from build123d import *

# Parameters (mm, degrees)
SKETCH016_W             = 35.6
SKETCH016_H             = 11.6
PAD009_DEPTH            = 0.8
SKETCH017_W             = 35.6
SKETCH017_H             = 11.6
SKETCH017_W_2           = 34
SKETCH017_H_2           = 10
PAD010_DEPTH            = 55.8
SKETCH018_W             = 6
SKETCH018_H             = 12
POCKET007_DEPTH         = 5.8
BODY005_PLACEMENT_ANGLE = 270


with BuildPart() as part:
    # Sketch016 → Pad009 (new body)
    with BuildSketch(Plane.XY):
        Rectangle(SKETCH016_W, SKETCH016_H)
    extrude(amount=PAD009_DEPTH)

    # Sketch017 → Pad010 (join)
    with BuildSketch(Plane.XY):
        Rectangle(SKETCH017_W, SKETCH017_H)
        Rectangle(SKETCH017_W_2, SKETCH017_H_2, mode=Mode.SUBTRACT)
    extrude(amount=PAD010_DEPTH)

    # Sketch018 (on Face5 of Pad010) → Pocket007 (cut)
    with BuildSketch(Plane.XZ.offset(5.8)):
        with Locations((14.8, 49.8)):
            Rectangle(SKETCH018_W, SKETCH018_H)
    extrude(amount=-POCKET007_DEPTH, mode=Mode.SUBTRACT)


with BuildPart() as part_1:
    # Body005 placement: moved
    add(part.part.moved(Location((-33.1, -35.587276, 51.887276))).rotate(Axis((-33.1, -35.587276, 51.887276), (1, 0, 0)), BODY005_PLACEMENT_ANGLE))


solid = part_1.part
Verification items for the finished model (mm, model axes). A direction names the side the tool comes from. Round coordinates to 2 decimals unless told otherwise and drop trailing zeros. Loops run counter-clockwise (first coordinate to the right, second up) from the corner with the lowest first, then second, coordinate; pieces in that order, holes last. Notation, with made-up numbers: (70.25, 39.5) - (85.25, 39.5) arc R31 ccw to (85.25, 74.5) - close; hole circle Ø8 at (66.5, 50). An arc over 180 degrees is marked (long way). Answer in a Markdown table with one row per item. Add a question column.
Q1. Section check B-B on y = -16.5. Enter the section's corners in (x, z).
Q2. Gauge pin test, flat ends, axial feed: pin 1 (2 mm diameter, centred on x = -35.5, z = 50.5, fed in from +Y); pin 2 (0.6 mm diameter, centred on y = 15.5, z = 57.5, fed in from +X). Record the tip position at first contact, or that the pin passes through.
Q3. Release check for a two-part mould opening along X. For faces 1 (the face through (-33, -35.587, 52)), 2 (the face through (-50.9, -8, 52)), 3 (the face through (-33, -8, 56.887)), 4 (the face through (-16.1, -8, 52)) record: pulls with the +X half, pulls with the -X half, needs draft (parallel to the pull), parting line crosses it, or undercut.
Q4. Tool access check on faces 5 (the face through (-33, -34.787, 52)), 6 (the face through (-35.8, 20.213, 46.7)). Record the directions out of +Z, -Z, +X, -X, +Y, -Y that give a thin tool (end or side, any length) a straight path to the whole face; none if there is none.
Q5. Section check A-A on x = -38.5. Enter the section's corners in (y, z), plus the area to 3 significant figures.
Q6. Section check D-D on y = 13. Enter the section's corners in (x, z), plus the area to 3 significant figures.
Q7. Material ranges on line 1 (Z direction, x = -38, y = -22); line 2 (X direction, y = -11, z = 48); line 3 (Y direction, x = -25.5, z = 47), recorded low to high.
Q8. Section check C-C on z = 50.75. Enter the section's corners in (x, y), plus the area to 3 significant figures.
Found:
| question | item | result |
|---|---|---|
| 1 | outline | (-50.9, 46.09) - (-15.3, 46.09) - (-15.3, 57.69) - (-50.9, 57.69) - close; hole (-50.1, 46.89) - (-16.1, 46.89) - (-16.1, 56.89) - (-50.1, 56.89) - close |
| 2 | pin 1 | stops at y = -34.79 |
| 2 | pin 2 | stops at x = -21.3 |
| 3 | face 1 | needs draft |
| 3 | face 2 | pulls with the -X half |
| 3 | face 3 | undercut |
| 3 | face 4 | undercut |
| 4 | face 5 | +Y |
| 4 | face 6 | +Z, -Z, +X, -X, +Y |
| 5 | outline | (-35.59, 46.09) - (20.21, 46.09) - (20.21, 46.89) - (-34.79, 46.89) - (-34.79, 56.89) - (20.21, 56.89) - (20.21, 57.69) - (-35.59, 57.69) - close |
| 5 | area | 97.3 mm² |
| 6 | outline | (-50.9, 46.09) - (-15.3, 46.09) - (-15.3, 51.89) - (-16.1, 51.89) - (-16.1, 46.89) - (-50.1, 46.89) - (-50.1, 56.89) - (-21.3, 56.89) - (-21.3, 57.69) - (-50.9, 57.69) - close |
| 6 | area | 64.2 mm² |
| 7 | line 1 | z = 46.09 to 46.89, 56.89 to 57.69 |
| 7 | line 2 | x = -50.9 to -50.1, -16.1 to -15.3 |
| 7 | line 3 | y = -35.59 to -34.79 |
| 8 | outline | (-50.9, -35.59) - (-15.3, -35.59) - (-15.3, 20.21) - (-16.1, 20.21) - (-16.1, -34.79) - (-50.1, -34.79) - (-50.1, 20.21) - (-50.9, 20.21) - close |
| 8 | area | 116 mm² |
